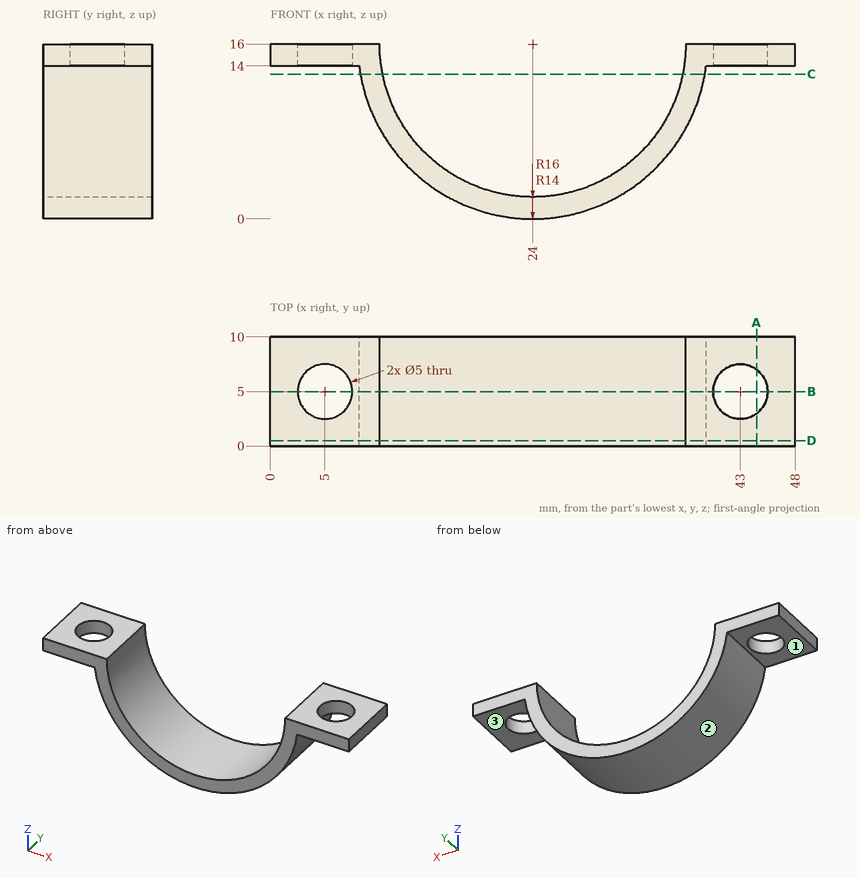
The figure shows three views and two pictorial views of one solid part (mm, origin at its lowest corner). Answer the questions. A direction names the side the tool comes from. Coordinates: 2 decimals unless noted, no trailing zeros. Order: outer loops, then holes, each group sorted by start corner. A loop starts at its lowest first (then second) coordinate and runs counter-clockwise, first axis right, second up. Notation, with made-up numbers: (53.25, -3.5) - (108.25, -3.5) arc R9 cw to (108.25, 2.5) - close; hole circle Ø1 at (-17.5, -27). An arc over 180 degrees is marked (long way). Answer as a JSON object with one key per item and string values.
1. Each of these flat-tipped pins is pushed along its axis until it touches: P1, Ø5, axis at x = 30, y = 8, coming from the -Z side; P2, Ø6, axis at y = 3.5, z = 11.5, coming from the +X side; P3, Ø6, axis at x = 43, y = 5, coming from the -Z side; P4, Ø3, axis at y = 5, z = 3.5, coming from the -X side. Where does it stop, or does it pass through?
Output values:
{"P1": "stops at z = 0.39", "P2": "stops at x = 48", "P3": "stops at z = 14", "P4": "stops at x = 12.38"}
2. A tool of negligible diameter and unlimited length cuts with its end or side. For the marked faces 1, 2 and 3, from which of +Z, -Z, +X, -X, +Y, -Y can it reach the whole face along a straight path? Write none if from no direction.
Output values:
{"face 1": "-Z, -X, +Y, -Y", "face 2": "-Z, +Y, -Y", "face 3": "-Z, +X, +Y, -Y"}
3. Find section B-B on y = 5. Determine the outline of the cut face in (x, z), plus the area to 3 significant figures.
Output values:
{"outline": "(0, 14) - (2.5, 14) - (2.5, 16) - (0, 16) - close; (7.5, 14) - (8.13, 14) arc R16 ccw to (39.87, 14) - (40.5, 14) - (40.5, 16) - (38, 16) arc R14 cw to (10, 16) - (7.5, 16) - close; (45.5, 14) - (48, 14) - (48, 16) - (45.5, 16) - close", "area": "106 mm²"}
4. Consider line 1 (Y direction, x = 43, z = 14.9); line 2 (X direction, y = 5.75, z = 15.25); line 3 (Z direction, x = 24.5, y = 9). Determine where each line is inside the solid, lowest interval first.
Output values:
{"line 1": "y = 0 to 2.5, 7.5 to 10", "line 2": "x = 0 to 2.62, 7.38 to 10.02, 37.98 to 40.62, 45.38 to 48", "line 3": "z = 0.01 to 2.01"}
5. Find section A-A on x = 44.5. Determine the outline of the cut face in (y, z), plus the area to 3 significant figures.
Output values:
{"outline": "(0, 14) - (3, 14) - (3, 16) - (0, 16) - close; (7, 14) - (10, 14) - (10, 16) - (7, 16) - close", "area": "12.0 mm²"}
6. Find section C-C on z = 13.25. Determine the outline of the cut face in (x, y), plus the area to 3 significant figures.
Output values:
{"outline": "(8.24, 0) - (10.27, 0) - (10.27, 10) - (8.24, 10) - close; (37.73, 0) - (39.76, 0) - (39.76, 10) - (37.73, 10) - close", "area": "40.7 mm²"}
7. Find section D-D on y = 0.5. Determine the outline of the cut face in (x, z), plus the area to 3 significant figures.
Output values:
{"outline": "(0, 14) - (8.13, 14) arc R16 ccw to (39.87, 14) - (48, 14) - (48, 16) - (38, 16) arc R14 cw to (10, 16) - (0, 16) - close", "area": "126 mm²"}
